from build123d import *

# Parameters (mm, degrees)
EXTRUDE_1_DEPTH     = 8
EXTRUDE_2_DEPTH     = 4.8
EXTRUDE_3_DEPTH     = 16
CUT_EXTRUDE_1_DEPTH = 15.747203125
CUT_EXTRUDE_START   = -4.8
SKETCH_5_R          = 0.35
CUT_EXTRUDE_2_DEPTH = 9.6
CHAMFER_1_SIZE      = 0.12
FILLET_1_R          = 0.2
FILLET_2_R          = 0.3
SKETCH_12_R         = 0.86
CUT_EXTRUDE_4_DEPTH = 1.5


with BuildPart() as part:
    # 草图1 → 凸台-拉伸1 (new, symmetric)
    with BuildSketch(Plane(origin=(0, 0, 0), x_dir=(0, 0, -1), z_dir=(1, 0, 0))):
        Polygon((-5.9, 3.7), (5.9, 3.7), (5.9, -0.3), (2.5, -0.3), (2.5, 1.8), (-2.5, 1.8), (-2.5, -0.3), (-5.9, -0.3), align=None)
    extrude(amount=EXTRUDE_1_DEPTH, both=True)

    # 草图2 → 凸台-拉伸2 (add, symmetric)
    with BuildSketch(Plane(origin=(0, 0, 0), x_dir=(0, 0, -1), z_dir=(1, 0, 0))):
        Polygon((6, 1.7), (6, 3.7), (5.5, 4.2), (-5.5, 4.2), (-6, 3.7), (-6, 1.7), (-5.9, 1.6), (-5.9, 3.7), (5.9, 3.7), (5.9, 1.6), align=None)
    extrude(amount=EXTRUDE_2_DEPTH, both=True)

    # 草图11 → 凸台-拉伸3 (add)
    with BuildSketch(Plane(origin=(8, 0, 0), x_dir=(0, 0, -1), z_dir=(1, 0, 0))):
        with BuildLine():
            Line((-2, 1.042), (-2.1, 1.042))
            ThreePointArc((-2.1, 1.042), (-2.260324923, 1.265329695), (-2.5, 1.4))
            Line((-2.5, 1.4), (-2.5, 0.184))
            ThreePointArc((-2.5, 0.184), (-2.260324923, 0.318670305), (-2.1, 0.542))
            Line((-2.1, 0.542), (-2, 0.542))
            ThreePointArc((-2, 0.542), (-1.75, 0.792), (-2, 1.042))
        make_face()
        with BuildLine():
            Line((2.5, 1.4), (2.5, 0.184))
            ThreePointArc((2.5, 0.184), (2.260324923, 0.318670305), (2.1, 0.542))
            Line((2.1, 0.542), (2, 0.542))
            ThreePointArc((2, 0.542), (1.75, 0.792), (2, 1.042))
            Line((2, 1.042), (2.1, 1.042))
            ThreePointArc((2.1, 1.042), (2.260324923, 1.265329695), (2.5, 1.4))
        make_face()
    extrude(amount=-EXTRUDE_3_DEPTH)

    # 草图3 → 切除-拉伸1 (cut, through all)
    with BuildSketch(Plane.ZY.offset(4.8)):
        Polygon((1.7, 4.2), (1.4, 3.9), (-1.4, 3.9), (-1.7, 4.2), align=None)
    extrude(amount=-CUT_EXTRUDE_1_DEPTH, mode=Mode.SUBTRACT)

    # 草图5 → 切除-拉伸2 (cut)
    with BuildSketch(Plane(origin=(0, 0, 0), x_dir=(0, 0, -1), z_dir=(1, 0, 0)).offset(CUT_EXTRUDE_START)):
        with Locations((-6.25, 2.7)):
            Circle(SKETCH_5_R)
    extrude(amount=CUT_EXTRUDE_2_DEPTH, mode=Mode.SUBTRACT)

    # 倒角1
    chamfer_1_edges = [part.edges().sort_by_distance(p)[0] for p in [
        (0, -0.3, 5.9),
        (6.4, 3.7, 5.9),
        (6.4, 3.7, -5.9),
        (0, -0.3, -5.9),
        (-6.4, 3.7, 5.9),
        (-6.4, 3.7, -5.9),
    ]]
    chamfer(chamfer_1_edges, length=CHAMFER_1_SIZE)

    # 圆角1
    fillet_1_edges = [part.edges().sort_by_distance(p)[0] for p in [
        (0, 0.184, -2.5),
        (0, 0.542, -2.1),
        (0, 1.042, -2.1),
        (0, 1.4, -2.5),
        (0, 0.184, 2.5),
        (0, 0.542, 2.1),
        (0, 1.042, 2.1),
        (0, 1.4, 2.5),
    ]]
    fillet(fillet_1_edges, radius=FILLET_1_R)

    # 圆角2
    # the kernel refuses this fillet: 0.3 mm, written as the material it adds along each edge
    with BuildSketch(Plane(origin=(8, 1.8, 2.5), x_dir=(0, -1, 0), z_dir=(-1, 0, 0))) as fillet_2_piece_1:
        with BuildLine():
            CenterArc((0.3, -0.298097301), FILLET_2_R, 96.456420664, 83.543579336)
            Line((0, -0.298097301), (-0.006, -0.298097301))
            Line((-0.006, -0.298097301), (-0.006, 0))
            Line((-0.006, 0), (0, 0.006))
            ThreePointArc((0, 0.006), (0.13313288, 0.006), (0.265591075, 0.005961946))
            Line((0.265591075, 0.005961946), (0.26626576, 0))
        make_face()
    extrude(amount=16)
    with BuildSketch(Plane(origin=(8, 1.8, -2.5), x_dir=(0, 0, 1), z_dir=(-1, 0, 0))) as fillet_2_piece_2:
        with BuildLine():
            CenterArc((0.298097301, -0.3), FILLET_2_R, 90, 83.543579336)
            Line((0, -0.26626576), (-0.005961946, -0.265591075))
            ThreePointArc((-0.005961946, -0.265591075), (-0.006, -0.13313288), (-0.006, 0))
            Line((-0.006, 0), (0, 0.006))
            Line((0, 0.006), (0.298097301, 0.006))
            Line((0.298097301, 0.006), (0.298097301, 0))
        make_face()
    extrude(amount=16)

    # 草图12 → 切除-拉伸4 (cut)
    with BuildSketch(Plane(origin=(0, 4.2, 0), x_dir=(1, 0, 0), z_dir=(0, 1, 0))):
        with Locations(Location((0, 4, 0), (0, 0, 270))):
            Circle(SKETCH_12_R)
        with Locations(Location((0, -4, 0), (0, 0, 270))):
            Circle(SKETCH_12_R)
    extrude(amount=-CUT_EXTRUDE_4_DEPTH, mode=Mode.SUBTRACT)


solid = part.part
Input: part model. Units: mm. Frame: model coordinates. A direction names the side the tool comes from. Coordinates: 2 decimals unless noted, no trailing zeros. Loops run counter-clockwise (first coordinate to the right, second up) from the corner with the lowest first, then second, coordinate; pieces in that order, holes last. Notation, with made-up numbers: (59, 4) -> (114, 4) arc R34 ccw to (114, 43) -> close; hole circle Ø8 at (62.25, 50.5). An arc over 180 degrees is marked (long way). Write each question's results on one line, items separated by ' | '. Start each with the question number.
Q1. Pin query (flat end, axial travel): pin 1 (1 mm diameter, centred on x = 6.5, z = 0.5, fed in from +Y); pin 2 (1.5 mm diameter, centred on x = 0, z = 4, fed in from +Y); pin 3 (2 mm diameter, centred on x = 0.5, z = -1, fed in from -Y). Return the tip coordinate at first contact, or that it passes through.
Q2. Section A-A, the plane z = -0.25. Return the cut outline in (x, y).
Q3. Ray query, line 1 (X direction, y = 3.45, z = 4); line 2 (X direction, y = 3.9, z = -4); line 3 (Y direction, x = 3, z = -2). Return the intervals inside material, ascending. Write a range as from..to.
Q4. Reachability of faces 1 (the flat face through (6, 3.7, 0)), 2 (the flat face through (0, 1, 5.9)), 3 (the flat face through (0, 2.7, -4)), 4 (the flat face through (-6, 3.7, 0)) from +Z, -Z, +X, -X, +Y, -Y: full face, straight path, thin tool, end or side. Return the list, or none.
Q5. Section B-B, the plane z = -4. Return the cut outline in (x, y).
Q6. Pull-direction query (X, two-part tool) for faces 5 (the cylindrical face through (0.26, 3.46, 4.82)), 6 (the flat face through (8, 2, 0)), 7 (the flat face through (0, 3, -6)), 8 (the flat face through (0, 2.7, 4)); classes: released by +X, released by -X, zero draft, split by the parting line, or undercut.
Found:
1) pin 1: y = 3.7 | pin 2: y = 2.7 | pin 3: y = 0.54
2) outline: (-8, 1.8) -> (8, 1.8) -> (8, 3.7) -> (4.8, 3.7) -> (4.8, 3.9) -> (-4.8, 3.9) -> (-4.8, 3.7) -> (-8, 3.7) -> close
3) line 1: -8..-0.86, 0.86..8 | line 2: -4.8..-0.86, 0.86..4.8 | line 3: 0.54..1.04, 1.8..4.2
4) face 1: +Z, -Z, +X, +Y | face 2: +Z, -Y | face 3: +Y | face 4: +Z, -Z, -X, +Y
5) outline: (-8, -0.3) -> (8, -0.3) -> (8, 3.7) -> (4.8, 3.7) -> (4.8, 4.2) -> (0.86, 4.2) -> (0.86, 2.7) -> (-0.86, 2.7) -> (-0.86, 4.2) -> (-4.8, 4.2) -> (-4.8, 3.7) -> (-8, 3.7) -> close
6) face 5: undercut | face 6: released by +X | face 7: zero draft | face 8: undercut
